Autodesk Inventor part; units mm, degrees
ref_plane "YZ Plane" through (0, 0, 0) normal (1, 0, 0) x (0, 1, 0)
ref_plane "XZ Plane" through (0, 0, 0) normal (0, 1, 0) x (-1, 0, 0)
ref_plane "XY Plane" through (0, 0, 0) normal (0, 0, 1) x (1, 0, 0)
sketch "スケッチ1" plane through (0, 0, 0) normal (0, 1, 0) x (-1, 0, 0)
  line L0 (-55, -7.5) -> (55, -7.5)
  line L1 (55, -7.5) -> (55, 7.5)
  line L2 (55, 7.5) -> (-55, 7.5)
  line L3 (-55, 7.5) -> (-55, -7.5)
  line L4 (-55, -7.5) -> (55, 7.5) construction
  line L5 (55, -7.5) -> (-55, 7.5) construction
  point P0 (0, 0)
  dimension "d0" = 110
  dimension "d1" = 15
extrude "押し出し1" add sketch "スケッチ1" along normal mid plane 5
sketch "スケッチ2" plane through (0, 2.5, 0) normal (0, 1, 0) x (1, 0, 0)
  circle A0 centre (50, 0) radius 1.45
  circle A1 centre (-50, 0) radius 1.45
  point P0 (0, 0)
  dimension "d4" = 2.9
  dimension "d5" = 2.9
extrude "押し出し2" cut sketch "スケッチ2" against normal blind 5
sketch "スケッチ3" plane through (0, 2.5, 0) normal (0, 1, 0) x (1, 0, 0)
  circle A0 centre (26, 0) radius 1.45
  circle A1 centre (-26, 0) radius 1.45
  point P0 (0, 0)
  dimension "d8" = 2.9
  dimension "d9" = 2.9
extrude "押し出し3" cut sketch "スケッチ3" against normal blind 5
sketch "スケッチ4" plane through (0, 2.5, 0) normal (0, 1, 0) x (1, 0, 0)
  line L0 (-6.25, 15) -> (6.25, 15)
  line L1 (6.25, 15) -> (6.25, -15)
  line L2 (6.25, -15) -> (-6.25, -15)
  line L3 (-6.25, -15) -> (-6.25, 15)
  line L4 (-6.25, 15) -> (6.25, -15) construction
  line L5 (6.25, 15) -> (-6.25, -15) construction
  point P0 (0, 0)
  dimension "d12" = 12.5
  dimension "d13" = 30
extrude "押し出し4" add sketch "スケッチ4" against normal blind 5
fillet "フィレット1" radius 8 4 edges at (6.25, 0, 7.5) (-6.25, 0, 7.5) (-6.25, 0, -7.5) (6.25, 0, -7.5)
sketch "スケッチ5" plane through (0, 2.5, 0) normal (0, 1, 0) x (1, 0, 0)
  circle A0 centre (0, -10) radius 2.25
  circle A1 centre (0, 10) radius 2.25
  point P0 (0, 0)
  dimension "d17" = 4.5
  dimension "d18" = 4.5
extrude "押し出し5" cut sketch "スケッチ5" against normal blind 5
properties part number "board2"
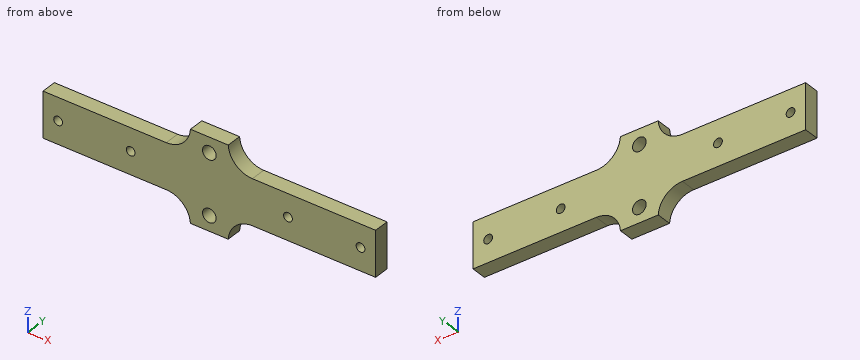
Design review of the part built by this model. Coordinates are the model's own, in mm. Round coordinates to 2 decimals unless told otherwise and drop trailing zeros. Write each loop counter-clockwise with the first axis right and the second up, starting at its lowest first coordinate (ties: lowest second). Pieces come first, ordered by that corner, then holes. Notation, with made-up numbers: (71, 83) -> (96, 83) arc R12 cw to (96, 106) -> close; hole circle Ø9 at (-36, -28). An arc over 180 degrees is marked (long way). Write item = value, one per line. Start each with the question number.
1) Take a section at A-A, the plane x = 50. State the section outline as (y, z) points, plus the area to 3 significant figures.
2) Take a section at C-C, the plane z = -10. State the section outline as (x, y) points.
3) Wall thickness on probe 1 along X at (y, z) = (0.95, 0); probe 2 along Z at (x, y) = (0, -0.8); probe 3 along Z at (x, y) = (26, -1.1): over which ranges is each line inside the solid? List them lowest first. Write a range as from..to.
4) Take a section at B-B, the plane y = 0.4. State the section outline as (x, z) points.
5) Clearance check with flat-ended pins moving along their axes: pin 1 (1.5 mm diameter, centred on x = -25.5, y = 0, fed in from -Z); pin 2 (1 mm diameter, centred on x = -20.5, y = 1.5, fed in from +Z). State where each tip first meets the part, or that it passes through.
6) Take a section at D-D, the plane x = -1. State the section outline as (y, z) points, plus the area to 3 significant figures.
Results list:
q1.outline = (-2.5, -7.5) -> (2.5, -7.5) -> (2.5, -1.45) -> (-2.5, -1.45) -> close; (-2.5, 1.45) -> (2.5, 1.45) -> (2.5, 7.5) -> (-2.5, 7.5) -> close
q1.area = 60.5 mm²
q2.outline = (-8.42, -2.5) -> (-2.25, -2.5) -> (-2.25, 2.5) -> (-8.42, 2.5) -> close; (2.25, -2.5) -> (8.42, -2.5) -> (8.42, 2.5) -> (2.25, 2.5) -> close
q3.probe_1 = -55..-51.45, -48.55..-27.45, -24.55..24.55, 27.45..48.55, 51.45..55
q3.probe_2 = -15..-12.25, -7.75..7.75, 12.25..15
q3.probe_3 = -7.5..-1.45, 1.45..7.5
q4.outline = (-55, -7.5) -> (-14.23, -7.5) arc R8 cw to (-6.25, -15) -> (6.25, -15) arc R8 cw to (14.23, -7.5) -> (55, -7.5) -> (55, 7.5) -> (14.23, 7.5) arc R8 cw to (6.25, 15) -> (-6.25, 15) arc R8 cw to (-14.23, 7.5) -> (-55, 7.5) -> close; hole circle Ø2.9 at (-50, 0); hole circle Ø2.9 at (-26, 0); hole circle Ø4.5 at (0, -10); hole circle Ø4.5 at (0, 10); hole circle Ø2.9 at (26, 0); hole circle Ø2.9 at (50, 0)
q5.pin_1 = -7.5
q5.pin_2 = 7.5
q6.outline = (-2.5, -15) -> (2.5, -15) -> (2.5, -12.02) -> (-2.5, -12.02) -> close; (-2.5, -7.98) -> (2.5, -7.98) -> (2.5, 7.98) -> (-2.5, 7.98) -> close; (-2.5, 12.02) -> (2.5, 12.02) -> (2.5, 15) -> (-2.5, 15) -> close
q6.area = 110 mm²
